Model file for the job. Use its own axes, mm. Face numbers are marked on the shaded views. A direction names the side the tool comes from. Give positions to 0.01 mm unless a question says otherwise; leave off trailing zeros. Loops run counter-clockwise (first coordinate to the right, second up) from the corner with the lowest first, then second, coordinate; pieces in that order, holes last. Notation, with made-up numbers: M 74.5,54.5 L 90.5,54.5 A21 ccw 90.5,72.5 Z; hole C 76,77.25 d10. An arc over 180 degrees is marked long. Answer in a Markdown table with one row per item.
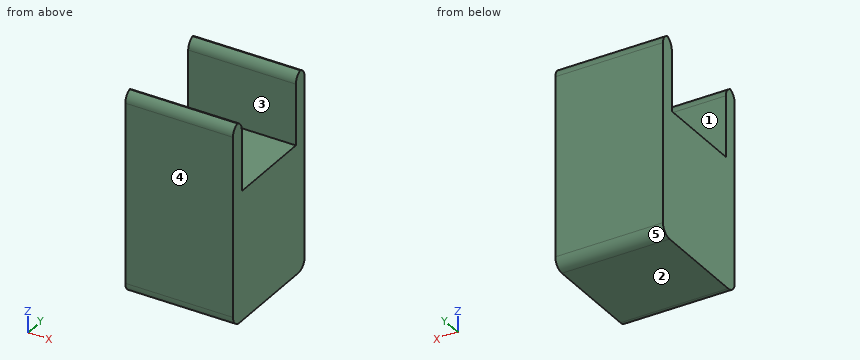
```python
from build123d import *

# Parameters (mm, degrees)
F1_DEPTH    = 7.5
F2_T1_DEPTH = 22.5


# Not quite as in the source:
# - a fillet or chamfer that OpenCascade refuses, or shapes differently, is made with other operations: its cross-section is extruded or revolved along the edge and cut away or added


with BuildPart() as f1:
    # F0 (on Right) → F1 (new body, symmetric)
    with BuildSketch(Plane.YZ):
        Polygon((6.15, 0), (0, 0), (-6.15, 0), (-6.15, 10), (-8.15, 10), (-8.15, -18), (0, -18), (8.15, -18), (8.15, 10), (6.15, 10), align=None)
    extrude(amount=F1_DEPTH, both=True)

    # F2: fillet of radius 1.5 on 6 edges, made by hand

    # F2_s2 → F2_t1 (cut)
    with BuildSketch(Plane.YZ.offset(-11.25)):
        with BuildLine():
            ThreePointArc((-8.15, 8.5), (-7.7106601718, 9.5606601718), (-6.65, 10))
            Line((-6.65, 10), (-8.15, 10))
            Line((-8.15, 10), (-8.15, 8.5))
        make_face()
        with BuildLine():
            ThreePointArc((-7.65, 10), (-6.5893398282, 9.5606601718), (-6.15, 8.5))
            Line((-6.15, 8.5), (-6.15, 10))
            Line((-6.15, 10), (-7.65, 10))
        make_face()
        with BuildLine():
            ThreePointArc((6.15, 8.5), (6.5893398282, 9.5606601718), (7.65, 10))
            Line((7.65, 10), (6.15, 10))
            Line((6.15, 10), (6.15, 8.5))
        make_face()
        with BuildLine():
            ThreePointArc((6.65, 10), (7.7106601718, 9.5606601718), (8.15, 8.5))
            Line((8.15, 8.5), (8.15, 10))
            Line((8.15, 10), (6.65, 10))
        make_face()
        with BuildLine():
            ThreePointArc((-6.65, -18), (-7.7106601718, -17.5606601718), (-8.15, -16.5))
            Line((-8.15, -16.5), (-8.15, -18))
            Line((-8.15, -18), (-6.65, -18))
        make_face()
        with BuildLine():
            ThreePointArc((8.15, -16.5), (7.7106601718, -17.5606601718), (6.65, -18))
            Line((6.65, -18), (8.15, -18))
            Line((8.15, -18), (8.15, -16.5))
        make_face()
    extrude(amount=F2_T1_DEPTH, mode=Mode.SUBTRACT)


solid = f1.part
```
Q1. Probe probe 1 along Y at (x, z) = (1.75, 5.5); probe 2 along Z at (x, y) = (7, 5). List the from-to ranges inside material, lowest first.
Reported:
| item | result |
|---|---|
| probe 1 | -8.15 to -6.15, 6.15 to 8.15 |
| probe 2 | -18 to 0 |
Q2. Mould opens along Y. For the marked faces 3, 4 and 5 say: released by +Y, released by -Y, zero draft, split by the parting line, or undercut.
Reported:
| item | result |
|---|---|
| face 3 | undercut |
| face 4 | released by -Y |
| face 5 | released by +Y |
Q3. Saw through at A-A (z = 7.25). Give the cut face in (x, y).
Reported:
| item | result |
|---|---|
| outline | M -7.5,-8.15 L 7.5,-8.15 L 7.5,-6.15 L -7.5,-6.15 Z; M -7.5,6.15 L 7.5,6.15 L 7.5,8.15 L -7.5,8.15 Z |
Q4. Drop a flat-ended pin along its axis: pin 1 (1.5 mm diameter, centred on y = -5, z = 5.5, fed in from -X). Give the stop position or say it passes through.
Reported:
| item | result |
|---|---|
| pin 1 | through |
Q5. Saw through at B-B (x = 2.75). Give the cut face in (y, z), and give its area (3 significant figures).
Reported:
| item | result |
|---|---|
| outline | M -8.15,-16.5 A1.5 ccw -6.65,-18 L 6.65,-18 A1.5 ccw 8.15,-16.5 L 8.15,8.5 A1.5 ccw 7.15,9.91 A1.5 ccw 6.15,8.5 L 6.15,0 L -6.15,0 L -6.15,8.5 A1.5 ccw -7.15,9.91 A1.5 ccw -8.15,8.5 Z |
| area | 331 mm² |
Q6. 3-axis set-ups, long thin cutter, end or side, ignore diameter. For the marked faces 1 and 2: which of +Z, -Z, +X, -X, +Y, -Y reach the whole face in a straight line?
Reported:
| item | result |
|---|---|
| face 1 | +Z, +X, -X |
| face 2 | -Z, +X, -X, +Y, -Y |
Q7. Saw through at C-C (y = 2.75). Give the cut face in (x, z), and give its area (3 significant figures).
Reported:
| item | result |
|---|---|
| outline | M -7.5,-18 L 7.5,-18 L 7.5,0 L -7.5,0 Z |
| area | 270 mm² |
